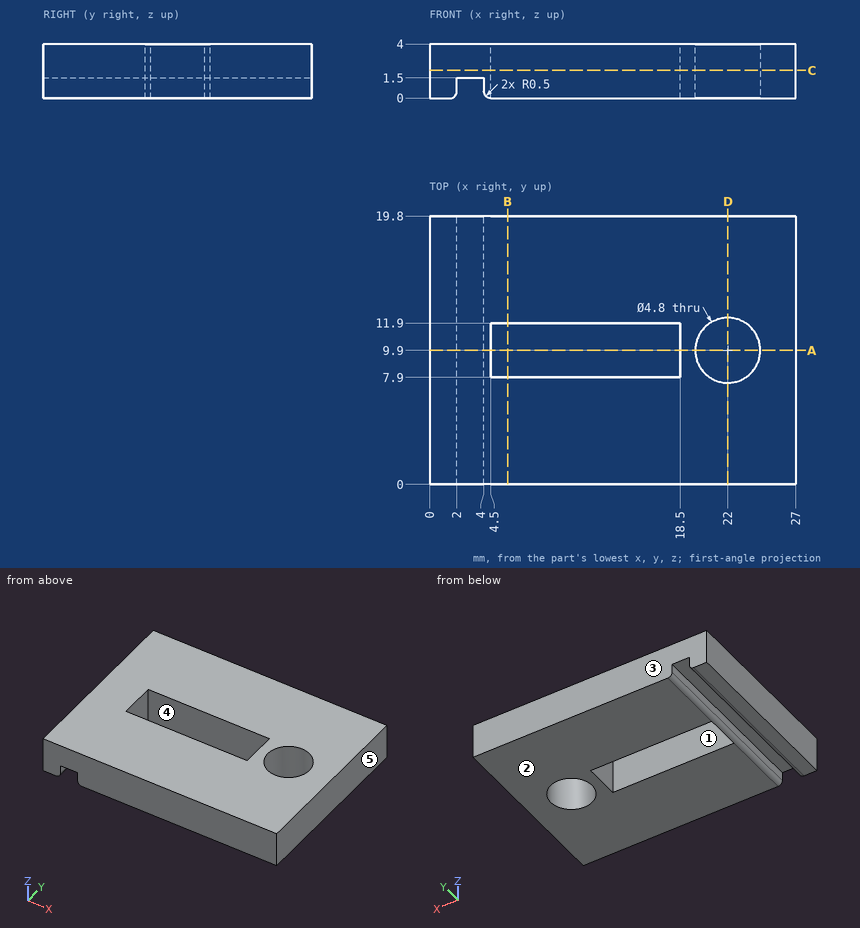
Answer from the drawing. Dimensions are ordinates in mm from the lowest x, y and z of the part. A direction names the side the tool comes from. Give positions to 0.01 mm unless a question says otherwise; leave off trailing zeros. Write each loop counter-clockwise with the first axis right and the second up, starting at its lowest first coordinate (ties: lowest second). Pieces come first, ordered by that corner, then holes. Notation, with made-up numbers: (-40, 33) -> (-20, 33) arc R15 ccw to (-20, 51) -> close; hole circle Ø10 at (-34, 32). An arc over 180 degrees is marked (long way). One line per question, with ' | ' between items. Start each with the question number.
1. Section A-A (y = 9.9) is taken. Determine the outline of the cut face in (x, z), plus the area to 3 significant figures.
2. Section B-B (x = 5.75) is taken. Determine the outline of the cut face in (y, z).
3. For the marked faces 1 and 2, determine the directions among +Z, -Z, +X, -X, +Y, -Y from which every point of the face is accessible in a straight line to the end or side of a thin tool.
4. Given pin 1 Ø7.5 at (x, y) = (22, 9.9) entering from -Z; pin 2 Ø0.6 at (x, y) = (2.5, 7.5) entering from -Z, each flat-ended and moving along its own axis, determine where each tip first touches the part or whether it passes through.
5. Section C-C (z = 2.05) is taken. Determine the outline of the cut face in (x, y).
6. Section D-D (x = 22) is taken. Determine the outline of the cut face in (y, z).
7. Find the intervals of material crossed by probe 1 along Y at (x, z) = (22, 2.75); probe 2 along X at (y, z) = (1.5, 1.35); probe 3 along Y at (x, z) = (5.5, 3.6), in increasing order.
8. For a pull along X with two mould halves and no side action, classify the marked faces 3, 4 and 5 as pulls with the +X half, pulls with the -X half, needs draft (parallel to the pull), parting line crosses it, or undercut.
Response values:
1) outline: (0, 0) -> (1.5, 0) arc R0.5 ccw to (2, 0.5) -> (2, 1.5) -> (4, 1.5) -> (4, 0.5) arc R0.5 ccw to (4.5, 0) -> (4.5, 4) -> (0, 4) -> close; (18.5, 0) -> (19.6, 0) -> (19.6, 4) -> (18.5, 4) -> close; (24.4, 0) -> (27, 0) -> (27, 4) -> (24.4, 4) -> close | area: 29.7 mm2
2) outline: (0, 0) -> (7.9, 0) -> (7.9, 4) -> (0, 4) -> close; (11.9, 0) -> (19.8, 0) -> (19.8, 4) -> (11.9, 4) -> close
3) face 1: +Z, -Z | face 2: -Z, +X, -X, +Y, -Y
4) pin 1: z = 0 | pin 2: z = 1.5
5) outline: (0, 0) -> (27, 0) -> (27, 19.8) -> (0, 19.8) -> close; hole (4.5, 7.9) -> (18.5, 7.9) -> (18.5, 11.9) -> (4.5, 11.9) -> close; hole circle Ø4.8 at (22, 9.9)
6) outline: (0, 0) -> (7.5, 0) -> (7.5, 4) -> (0, 4) -> close; (12.3, 0) -> (19.8, 0) -> (19.8, 4) -> (12.3, 4) -> close
7) probe 1: 0 to 7.5, 12.3 to 19.8 | probe 2: 0 to 2, 4 to 27 | probe 3: 0 to 7.9, 11.9 to 19.8
8) face 3: needs draft | face 4: undercut | face 5: pulls with the +X half
